Verification items for the finished model (mm, model axes). A direction names the side the tool comes from. Coordinates: 2 decimals unless noted, no trailing zeros. Write each loop counter-clockwise with the first axis right and the second up, starting at its lowest first coordinate (ties: lowest second). Pieces come first, ordered by that corner, then holes. Notation, with made-up numbers: (24, 47.25) -> (82, 47.25) arc R16 cw to (82, 67.25) -> close; hole circle Ø5 at (49, 89.25). An arc over 180 degrees is marked (long way). Answer in a Markdown table with one row per item.
```python
from build123d import *

# Parameters (mm, degrees)
SKETCH1_R           = 1.5
SKETCH1_R_2         = 3.375
BOSS_EXTRUDE1_DEPTH = 3


with BuildPart() as part:
    # Sketch1 → Boss-Extrude1 (new body)
    with BuildSketch(Plane.XY):
        Polygon((213, -20.5), (213, 2), (216, 2), (216, 24.5), (213, 24.5), (213, 47), (128, 47), (128, 44), (78, 44), (78, 47), (-2, 47), (-2, 24.5), (-5, 24.5), (-5, 2), (-2, 2), (-2, -20.5), (-5, -20.5), (-5, -43), (-2, -43), (78, -43), (78, -40), (128, -40), (128, -43), (213, -43), (216, -43), (216, -20.5), align=None)
        with Locations((8, 35.117670932)):
            Circle(SKETCH1_R, mode=Mode.SUBTRACT)
        with Locations((8, 3)):
            Circle(SKETCH1_R, mode=Mode.SUBTRACT)
        with Locations((203, 3)):
            Circle(SKETCH1_R, mode=Mode.SUBTRACT)
        with Locations((203, 35.117670932)):
            Circle(SKETCH1_R, mode=Mode.SUBTRACT)
        with Locations((72.75, 27.117670932)):
            Circle(SKETCH1_R_2, mode=Mode.SUBTRACT)
        with Locations((72.75, 11)):
            Circle(SKETCH1_R_2, mode=Mode.SUBTRACT)
        with Locations((138.25, 27.117670932)):
            Circle(SKETCH1_R_2, mode=Mode.SUBTRACT)
        with Locations((138.25, 11)):
            Circle(SKETCH1_R_2, mode=Mode.SUBTRACT)
        with BuildLine():
            Line((15, 10), (15, 28.117670932))
            ThreePointArc((15, 28.117670932), (26, 33.308835466), (37, 28.117670932))
            Line((37, 28.117670932), (37, 10))
            ThreePointArc((37, 10), (26, 4.808835466), (15, 10))
        make_face(mode=Mode.SUBTRACT)
        with BuildLine():
            Line((43, 10), (43, 28.117670932))
            ThreePointArc((43, 28.117670932), (54, 33.308835466), (65, 28.117670932))
            Line((65, 28.117670932), (65, 10))
            ThreePointArc((65, 10), (54, 4.808835466), (43, 10))
        make_face(mode=Mode.SUBTRACT)
        with BuildLine():
            Line((80.5, 10), (80.5, 28.117670932))
            ThreePointArc((80.5, 28.117670932), (91.5, 33.308835466), (102.5, 28.117670932))
            Line((102.5, 28.117670932), (102.5, 10))
            ThreePointArc((102.5, 10), (91.5, 4.808835466), (80.5, 10))
        make_face(mode=Mode.SUBTRACT)
        with BuildLine():
            Line((108.5, 10), (108.5, 28.117670932))
            ThreePointArc((108.5, 28.117670932), (119.5, 33.308835466), (130.5, 28.117670932))
            Line((130.5, 28.117670932), (130.5, 10))
            ThreePointArc((130.5, 10), (119.5, 4.808835466), (108.5, 10))
        make_face(mode=Mode.SUBTRACT)
        with BuildLine():
            Line((146, 10), (146, 28.117670932))
            ThreePointArc((146, 28.117670932), (157, 33.308835466), (168, 28.117670932))
            Line((168, 28.117670932), (168, 10))
            ThreePointArc((168, 10), (157, 4.808835466), (146, 10))
        make_face(mode=Mode.SUBTRACT)
        with BuildLine():
            Line((174, 10), (174, 28.117670932))
            ThreePointArc((174, 28.117670932), (185, 33.308835466), (196, 28.117670932))
            Line((196, 28.117670932), (196, 10))
            ThreePointArc((196, 10), (185, 4.808835466), (174, 10))
        make_face(mode=Mode.SUBTRACT)
    extrude(amount=BOSS_EXTRUDE1_DEPTH)


solid = part.part
```
1. Sectioned sample at D-D, the plane x = 186. Record the cut outline in (y, z).
Findings below:
| item | result |
|---|---|
| outline | (-43, 0) -> (4.84, 0) -> (4.84, 3) -> (-43, 3) -> close; (33.27, 0) -> (47, 0) -> (47, 3) -> (33.27, 3) -> close |
2. Access from +Z, -Z, +X, -X, +Y, -Y to the whole of each face (thin tool, end or side, straight path). Record for faces 4 (the face through (184.824, 33.308, 1.479)), 5 (the face through (104, 3, 3)).
Findings below:
| item | result |
|---|---|
| face 4 | +Z, -Z |
| face 5 | +Z, +X, -X, +Y, -Y |
3. Release check for a two-part mould opening along Y. For faces 1 (the face through (141.47, 12.01, 1.48)), 2 (the face through (104, 3, 0)), 3 (the face through (119.68, 4.81, 1.48)) record: released by +Y, released by -Y, zero draft, split by the parting line, or undercut.
Findings below:
| item | result |
|---|---|
| face 1 | undercut |
| face 2 | zero draft |
| face 3 | undercut |
4. Sectioned sample at B-B, the plane y = 18.5. Record the cut outline in (x, z), and give its area (3 significant figures).
Findings below:
| item | result |
|---|---|
| outline | (-5, 0) -> (15, 0) -> (15, 3) -> (-5, 3) -> close; (37, 0) -> (43, 0) -> (43, 3) -> (37, 3) -> close; (65, 0) -> (80.5, 0) -> (80.5, 3) -> (65, 3) -> close; (102.5, 0) -> (108.5, 0) -> (108.5, 3) -> (102.5, 3) -> close; (130.5, 0) -> (146, 0) -> (146, 3) -> (130.5, 3) -> close; (168, 0) -> (174, 0) -> (174, 3) -> (168, 3) -> close; (196, 0) -> (216, 0) -> (216, 3) -> (196, 3) -> close |
| area | 267 mm² |
5. Go/stop test with flat-tipped pins: pin 1 (6 mm diameter, centred on x = 138.25, y = 11, fed in from +Z); pin 2 (1 mm diameter, centred on x = 126, z = 2, fed in from +Y); pin 3 (0.9 mm diameter, centred on x = -3.5, z = 2, fed in from +Y). Record where each tip stops, or that it passes through.
Findings below:
| item | result |
|---|---|
| pin 1 | passes through |
| pin 2 | stops at y = 44 |
| pin 3 | stops at y = 24.5 |
6. Sectioned sample at C-C, the plane x = 29.5. Record the cut outline in (y, z).
Findings below:
| item | result |
|---|---|
| outline | (-43, 0) -> (5.25, 0) -> (5.25, 3) -> (-43, 3) -> close; (32.87, 0) -> (47, 0) -> (47, 3) -> (32.87, 3) -> close |
7. Material ranges on probe 1 along Y at (x, z) = (8, 1.8); probe 2 along Y at (x, z) = (72.75, 0.9) (3 decimals); probe 3 along Y at (x, z) = (124.5, 0.8), recorded low to high. Write a range as from..to.
Findings below:
| item | result |
|---|---|
| probe 1 | y = -43..1.5, 4.5..33.62, 36.62..47 |
| probe 2 | y = -43..7.625, 14.375..23.743, 30.493..47 |
| probe 3 | y = -40..5.71, 32.4..44 |
8. Sectioned sample at A-A, the plane x = 138.25. Record the cut outline in (y, z) (3 decimals).
Findings below:
| item | result |
|---|---|
| outline | (-43, 0) -> (7.625, 0) -> (7.625, 3) -> (-43, 3) -> close; (14.375, 0) -> (23.743, 0) -> (23.743, 3) -> (14.375, 3) -> close; (30.493, 0) -> (47, 0) -> (47, 3) -> (30.493, 3) -> close |
